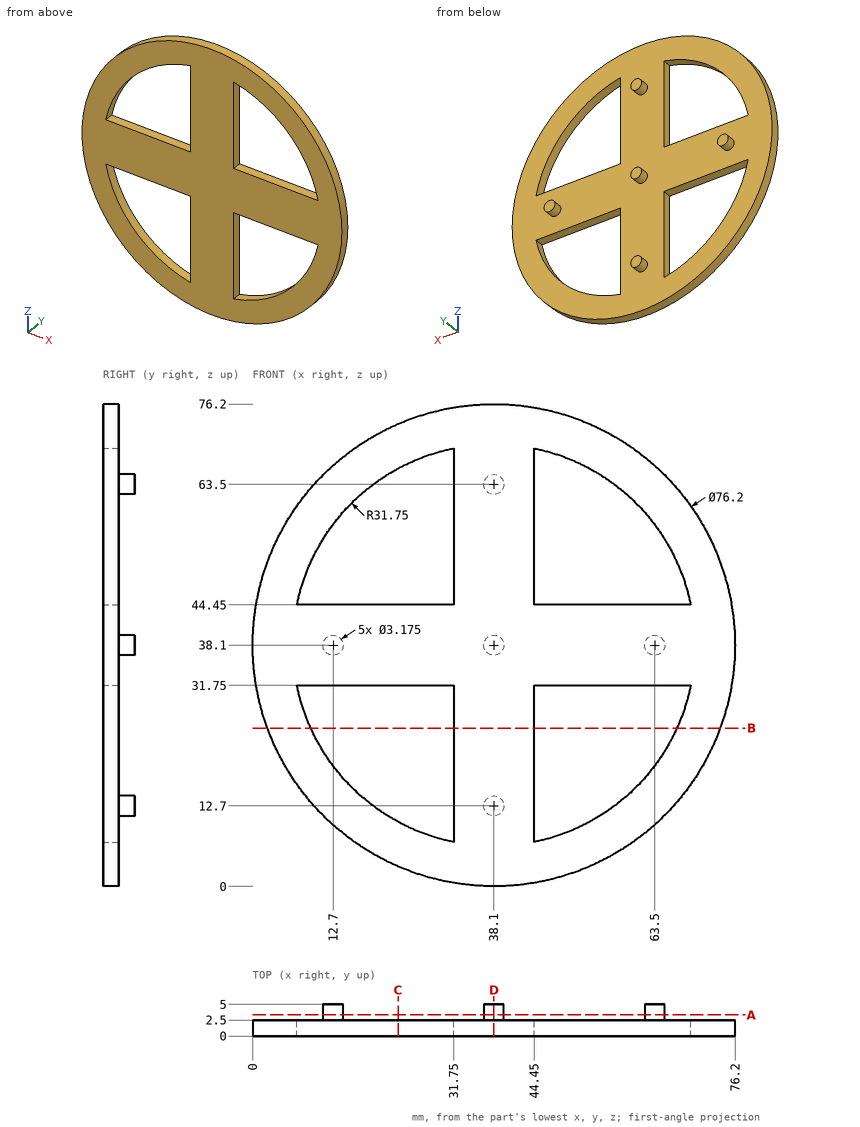
Geometry check sheet. Reference: drawing and pictorial views, mm from the part's lowest x, y, z. Coordinates: 2 decimals unless noted, no trailing zeros. Order: outer loops, then holes, each group sorted by start corner. A loop starts at its lowest first (then second) coordinate and runs counter-clockwise, first axis right, second up.
Item 1: Section check A-A (y = 3.35). Enter the section's corners in (x, z) (1 decimal).
Item 2: Scan lines: line 1 along Z through (x, y) = (67, 2); line 2 along X through (y, z) = (1.65, 60); line 3 along Z through (x, y) = (30, 1.95). Record each from-to range of solid material in increasing order.
Item 3: Section check B-B (z = 25). Enter the section's corners in (x, y), plus the area to 3 significant figures.
Item 4: Section check D-D (x = 38.1). Enter the section's corners in (y, z).
Item 5: Section check C-C (x = 23). Enter the section's corners in (y, z).
Item 6: Depth check by flat-ended pin: pin 1 (2 mm diameter, centred on y = 1.5, z = 49, fed in from -X); pin 2 (1.2 mm diameter, centred on y = 1, z = 55, fed in from -X); pin 3 (2 mm diameter, centred on y = 1.5, z = 13.5, fed in from +X); pin 4 (2 mm diameter, centred on x = 15.5, z = 30, fed in from +Y). Enter the tip coordinate at first touch or a pass-through.
Check sheet entries:
1. outline: circle Ø3.2 at (12.7, 38.1); circle Ø3.2 at (38.1, 12.7); circle Ø3.2 at (38.1, 38.1); circle Ø3.2 at (38.1, 63.5); circle Ø3.2 at (63.5, 38.1)
2. line 1: z = 13.27 to 24.95, 31.75 to 44.45, 51.25 to 62.93
2. line 2: x = 6.92 to 15.11, 31.75 to 44.45, 61.09 to 69.28
2. line 3: z = 0.87 to 7.4, 31.75 to 44.45, 68.8 to 75.33
3. outline: (2.32, 0) - (9.18, 0) - (9.18, 2.5) - (2.32, 2.5) - close; (31.75, 0) - (44.45, 0) - (44.45, 2.5) - (31.75, 2.5) - close; (67.02, 0) - (73.88, 0) - (73.88, 2.5) - (67.02, 2.5) - close
3. area: 66.0 mm2
4. outline: (0, 0) - (2.5, 0) - (2.5, 11.11) - (5, 11.11) - (5, 14.29) - (2.5, 14.29) - (2.5, 36.51) - (5, 36.51) - (5, 39.69) - (2.5, 39.69) - (2.5, 61.91) - (5, 61.91) - (5, 65.09) - (2.5, 65.09) - (2.5, 76.2) - (0, 76.2) - close
5. outline: (0, 3.12) - (2.5, 3.12) - (2.5, 10.17) - (0, 10.17) - close; (0, 31.75) - (2.5, 31.75) - (2.5, 44.45) - (0, 44.45) - close; (0, 66.03) - (2.5, 66.03) - (2.5, 73.08) - (0, 73.08) - close
6. pin 1: stops at x = 1.31
6. pin 2: stops at x = 3.66
6. pin 3: stops at x = 68.01
6. pin 4: passes through
